Verification items for the finished model (mm, model axes). Face numbers are marked on the shaded views. Coordinates: 2 decimals unless noted, no trailing zeros. Order: outer loops, then holes, each group sorted by start corner. A loop starts at its lowest first (then second) coordinate and runs counter-clockwise, first axis right, second up. Notation, with made-up numbers: M 49,59 L 81,59 A28 cw 81,98 Z; hole C 70.5,13.25 d1. An arc over 180 degrees is marked long. Answer as a JSON object with one key per item and string values. Group by question number.
(1) Material ranges on line 1 (X direction, y = -1.8, z = -10); line 2 (Z direction, x = -24, y = -0.8); line 3 (X direction, y = -2.2, z = -1.5), recorded low to high.
(2) Mould release check, pull along Y, two halves, no side actions. Record for the marked faces 1 and 2: released by +Y, released by -Y, zero draft, split by the parting line, or undercut.
(3) Cross-section at B-B (z = 9.5). Enter the section's corners in (x, y).
(4) Gauge pin test, flat ends, axial feed: pin 1 Ø1 at (x, y) = (32, -2.5) entering from -Z; pin 2 Ø1.5 at (y, z) = (-1.5, -13.5) entering from -X; pin 3 Ø1.5 at (y, z) = (-2, 14) entering from +X; pin 4 Ø4 at (x, z) = (3.5, -1) entering from +Y. Record the tip position at first contact, or that the pin passes through.
(5) Cross-section at A-A (z = -8). Enter the section's corners in (x, y).
(6) Cross-section at D-D (x = 32). Enter the section's corners in (y, z), plus the area to 3 significant figures.
(7) Cross-section at C-C (y = -1). Count the separate pieces of the cut face and the enclosed holes in it, plus the area to 3 significant figures.
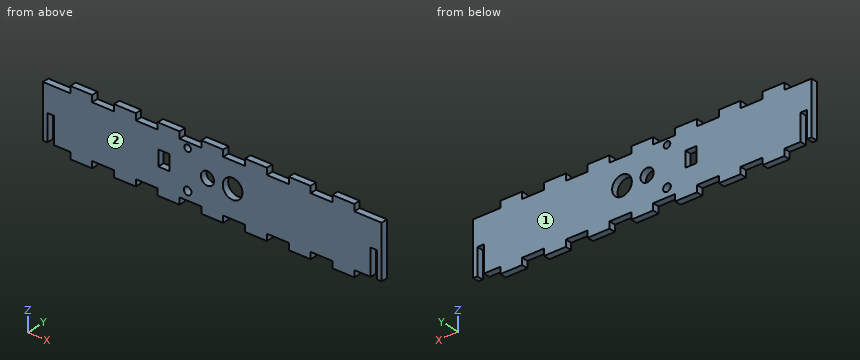
from build123d import *

# Parameters (mm, degrees)
F0_W     = 151
F0_H     = 30
F1_DEPTH = 3
F2_W     = 5
F2_H     = 3
F2_W_2   = 6.4484283328
F2_W_3   = 10
F2_W_4   = 3.5515716672
F2_R     = 4.5
F2_R_2   = 1.5
F2_R_3   = 1.75
F2_R_4   = 3
F2_H_2   = 7
F3_DEPTH = 25
F4_DEPTH = 2
F5_DEPTH = 2
F6_W     = 3
F6_H     = 12
F7_DEPTH = 25


with BuildPart() as f1:
    # F0 (on Front) → F1 (new body)
    with BuildSketch(Plane.XZ):
        Rectangle(F0_W, F0_H)
    extrude(amount=F1_DEPTH)

    # F2 (on face) → F3 (cut)
    with BuildSketch(Plane.XZ.offset(3)):
        with Locations((-72.5, -13.5)):
            Rectangle(F2_W, F2_H)
        with Locations((-78.2242141664, -13.5)):
            Rectangle(F2_W_2, F2_H)
        with Locations((-67.5, -13.5)):
            Rectangle(F2_W, F2_H)
        with Locations((-72.5, 13.5)):
            Rectangle(F2_W, F2_H)
        with Locations((-78.2242141664, 13.5)):
            Rectangle(F2_W_2, F2_H)
        with Locations((-67.5, 13.5)):
            Rectangle(F2_W, F2_H)
        with Locations((-50, -13.5)):
            Rectangle(F2_W_3, F2_H)
        with Locations((-50, 13.5)):
            Rectangle(F2_W_3, F2_H)
        with Locations((-30, -13.5)):
            Rectangle(F2_W_3, F2_H)
        with Locations((-30, 13.5)):
            Rectangle(F2_W_3, F2_H)
        with Locations((-10, -13.5)):
            Rectangle(F2_W_3, F2_H)
        with Locations((-10, 13.5)):
            Rectangle(F2_W_3, F2_H)
        with Locations((10, -13.5)):
            Rectangle(F2_W_3, F2_H)
        with Locations((10, 13.5)):
            Rectangle(F2_W_3, F2_H)
        with Locations((30, -13.5)):
            Rectangle(F2_W_3, F2_H)
        with Locations((30, 13.5)):
            Rectangle(F2_W_3, F2_H)
        with Locations((50, -13.5)):
            Rectangle(F2_W_3, F2_H)
        with Locations((50, 13.5)):
            Rectangle(F2_W_3, F2_H)
        with Locations((66.7757858336, -13.5)):
            Rectangle(F2_W_4, F2_H)
        with Locations((71.7757858336, -13.5)):
            Rectangle(F2_W_2, F2_H)
        with Locations((77.5, -13.5)):
            Rectangle(F2_W, F2_H)
        with Locations((66.7757858336, 13.5)):
            Rectangle(F2_W_4, F2_H)
        with Locations((71.7757858336, 13.5)):
            Rectangle(F2_W_2, F2_H)
        with Locations((77.5, 13.5)):
            Rectangle(F2_W, F2_H)
        with Locations((9.2957439325, 0.5)):
            Circle(F2_R)
        with Locations((-11.3042560675, 9.5)):
            Circle(F2_R_2)
        with Locations((-11.3042560675, -8)):
            Circle(F2_R_3)
        with Locations((-2.2042560675, 0.5)):
            Circle(F2_R_4)
        with Locations((-22.2042560675, 0.5)):
            Rectangle(F2_W, F2_H_2)
    extrude(amount=-F3_DEPTH, mode=Mode.SUBTRACT)

    # F4 (add): a face of the model
    f4_faces = [f1.faces().sort_by_distance(p)[0] for p in [
        (75.5, -1.5, 0),
    ]]
    extrude(f4_faces, amount=F4_DEPTH)

    # F5 (add): a face of the model
    f5_faces = [f1.faces().sort_by_distance(p)[0] for p in [
        (-75.5, -1.5, 0),
    ]]
    extrude(f5_faces, amount=F5_DEPTH)

    # F6 (on face) → F7 (cut)
    with BuildSketch(Plane(origin=(0, 0, 0), x_dir=(-1, 0, 0), z_dir=(0, 1, 0))):
        with Locations((74, -6)):
            Rectangle(F6_W, F6_H)
        with Locations((-74, -6)):
            Rectangle(F6_W, F6_H)
    extrude(amount=-F7_DEPTH, mode=Mode.SUBTRACT)


solid = f1.part
Taken from the geometry:
{
 "1": {"line 1": "x = -77.5 to -75.5, -72.5 to 72.5, 75.5 to 77.5", "line 2": "z = -15 to -3, 4 to 15", "line 3": "x = -77.5 to -75.5, -72.5 to -24.7, -19.7 to -4.44, 0.03 to 5.26, 13.33 to 72.5, 75.5 to 77.5"},
 "2": {"face 1": "released by +Y", "face 2": "released by -Y"},
 "3": {"outline": "M -77.5,-3 L -12.8,-3 L -12.8,0 L -77.5,0 Z; M -9.8,-3 L 77.5,-3 L 77.5,0 L -9.8,0 Z"},
 "4": {"pin 1": "stops at z = -12", "pin 2": "stops at x = -65", "pin 3": "stops at x = 65", "pin 4": "stops at y = 0"},
 "5": {"outline": "M -77.5,-3 L -75.5,-3 L -75.5,0 L -77.5,0 Z; M -72.5,-3 L -13.05,-3 L -13.05,0 L -72.5,0 Z; M -9.55,-3 L 72.5,-3 L 72.5,0 L -9.55,0 Z; M 75.5,-3 L 77.5,-3 L 77.5,0 L 75.5,0 Z"},
 "6": {"outline": "M -3,-12 L 0,-12 L 0,12 L -3,12 Z", "area": "72.0 mm²"},
 "7": {"separate pieces": "1", "enclosed holes": "5", "area": "3,920 mm²"}
}
